Input: dimensioned drawing with shaded views. Units: mm. Origin: part minimum x, y, z. A direction names the side the tool comes from. Coordinates: 2 decimals unless noted, no trailing zeros. Order: outer loops, then holes, each group sorted by start corner. A loop starts at its lowest first (then second) coordinate and runs counter-clockwise, first axis right, second up. Notation, with made-up numbers: (14.25, -5) - (23.25, -5) arc R26 ccw to (23.25, 26) - close; hole circle Ø4 at (73.5, 5). An arc over 180 degrees is marked (long way). Answer as CSV lines item,"result". Start each with the question number.
Item 1: Section C-C (x = 2.45). State how many separate pieces and enclosed holes the cut face has, and give its area (3 significant figures).
Item 2: Section A-A (y = 4.5). Output: boundary loops of the cut face in (x, z).
Item 3: Section D-D (z = 3.8). Output: boundary loops of the cut face in (x, y).
Item 4: First-contact query: pin 1 (1 mm diameter, centred on y = 13.5, z = 14.5, fed in from -X); pin 2 (1.5 mm diameter, centred on x = 1, z = 17.5, fed in from +Y); pin 3 (1 mm diameter, centred on x = 2.5, y = 20, fed in from +Z); pin 4 (1.5 mm diameter, centred on x = 1.5, y = 1.5, fed in from +Z). Flat tips, straight axial feed; report the tip coordinate or a pass-through.
Item 5: Access query for the marked faces 1, 2, 3, 4 and 5. Directions: +Z, -Z, +X, -X, +Y, -Y. A direction counts if a zero-diameter tool reaches every point of the face in a straight line with its end or side. Return the directions, or none.
Item 6: Section B-B (z = 13.8). Output: boundary loops of the cut face in (x, y), and give its area (3 significant figures).
Item 7: Material intervals for line 1 along Y through (x, z) = (1.5, 3.75) (1 decimal); line 2 along Y through (x, z) = (1.7, 12.75) (1 decimal); line 3 along Y through (x, z) = (1, 17.5), sorted ascending.
Item 8: Draft query along Y for the marked faces 6, 7, 8 and 9. Return one class per face: +Y half, -Y half, draft (parallel to the pull), parting line (faces both ways), or undercut.
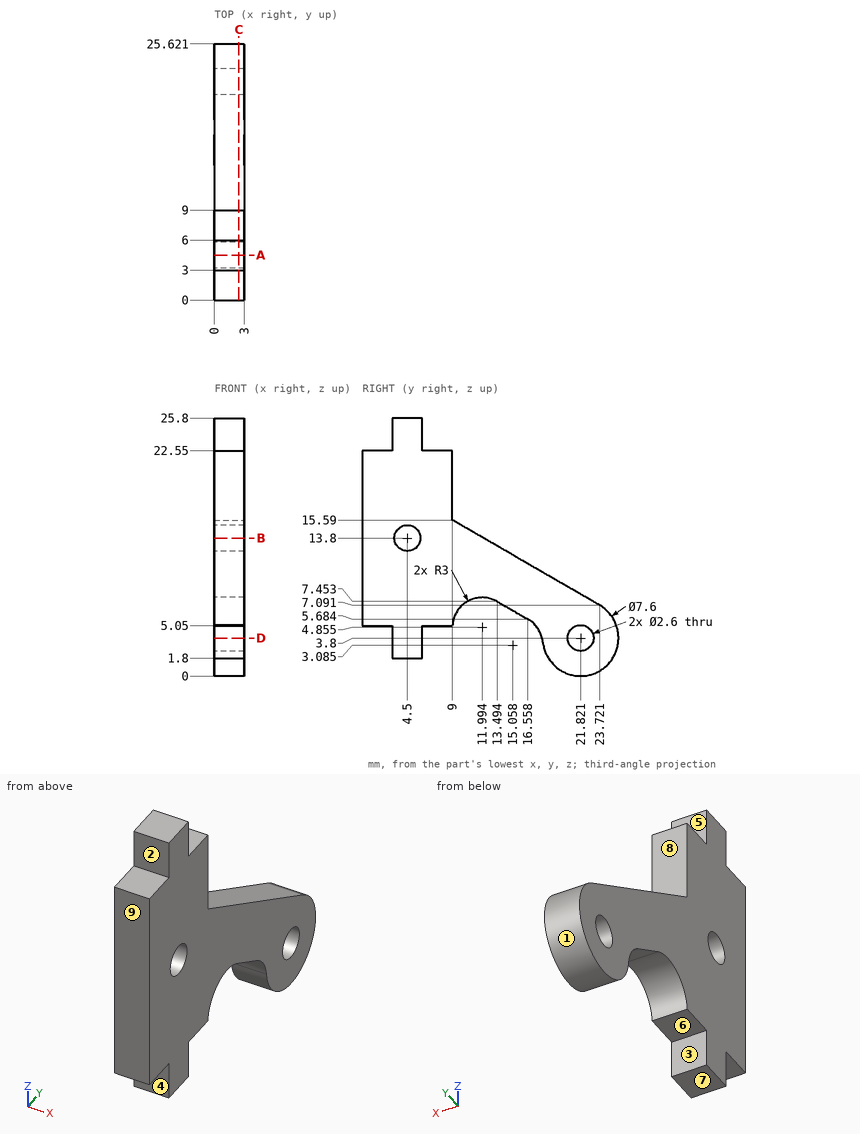
Determined:
1,separate pieces,"1"
1,enclosed holes,"2"
1,area,"278 mm^2"
2,outline,"(0, 1.8) - (3, 1.8) - (3, 12.5) - (0, 12.5) - close; (0, 15.1) - (3, 15.1) - (3, 25.8) - (0, 25.8) - close"
3,outline,"(0, 3) - (3, 3) - (3, 6) - (0, 6) - close; (0, 17.97) - (3, 17.97) - (3, 20.52) - (0, 20.52) - close; (0, 23.12) - (3, 23.12) - (3, 25.62) - (0, 25.62) - close"
4,pin 1,"passes through"
4,pin 2,"stops at y = 9"
4,pin 3,"stops at z = 9.53"
4,pin 4,"stops at z = 22.55"
5,face 1,"+X, -X"
5,face 2,"+Z, +X, -X, -Y"
5,face 3,"-Z, +X, -X"
5,face 4,"-Z, +X, -X, -Y"
5,face 5,"+Z, +X, -X, +Y"
6,outline,"(0, 0) - (3, 0) - (3, 3.2) - (0, 3.2) - close; (0, 5.8) - (3, 5.8) - (3, 12.1) - (0, 12.1) - close"
6,area,"28.5 mm^2"
7,line 1,"y = 3 to 6, 18 to 20.5, 23.1 to 25.6"
7,line 2,"y = 0 to 3.7, 5.3 to 13.9"
7,line 3,"y = 0 to 9"
8,face 6,"undercut"
8,face 7,"draft"
8,face 8,"+Y half"
8,face 9,"-Y half"
